```python
from build123d import *

# Parameters (mm, degrees)
PAD_DEPTH    = 39
PAD001_DEPTH = 35
SKETCH002_R  = 2.75
HOLE_DEPTH   = 10
HOLE_TIPS_R  = 2.75


with BuildPart() as part:
    # Sketch → Pad (new body)
    with BuildSketch(Plane.XZ):
        with BuildLine():
            ThreePointArc((8.810546, -10.5), (0, 13.706777), (-8.810546, -10.5))
            Line((-19.5, -10.5), (-8.810546, -10.5))
            Line((-19.5, -10.5), (-19.5, 8.5))
            Line((-19.5, 8.5), (-20.5, 8.5))
            Line((-20.5, 8.5), (-20.5, 17.5))
            Line((-20.5, 17.5), (-8.5, 17.5))
            Line((-8.5, 17.5), (-8.5, 16.5))
            Line((-8.5, 16.5), (8.5, 16.5))
            Line((8.5, 16.5), (8.5, 17.5))
            Line((8.5, 17.5), (20.5, 17.5))
            Line((20.5, 8.5), (20.5, 17.5))
            Line((19.5, 8.5), (20.5, 8.5))
            Line((19.5, -10.5), (19.5, 8.5))
            Line((8.810546, -10.5), (19.5, -10.5))
        make_face()
    extrude(amount=PAD_DEPTH)

    # Sketch001 (on DatumPlane) → Pad001 (join)
    with BuildSketch(Plane.XZ.offset(37)):
        with BuildLine():
            ThreePointArc((8.809308, -10.501039), (0.000808, 13.706777), (-8.810546, -10.5))
            Line((-7.713451, -9.192533), (-8.810546, -10.5))
            ThreePointArc((7.713451, -9.192533), (0, 12), (-7.713451, -9.192533))
            Line((7.713451, -9.192533), (8.809308, -10.501039))
        make_face()
    extrude(amount=-PAD001_DEPTH)

    # Sketch002 (on Face13 of Pad001) → Hole (cut)
    with BuildSketch(Plane(origin=(0, 0, 17.5), x_dir=(-1, 0, 0), z_dir=(0, 0, 1))):
        with Locations((-14, 32.5)):
            Circle(SKETCH002_R)
        with Locations((14, 32.5)):
            Circle(SKETCH002_R)
        with Locations((14, 6.5)):
            Circle(SKETCH002_R)
        with Locations((-14, 6.5)):
            Circle(SKETCH002_R)
    extrude(amount=-HOLE_DEPTH, mode=Mode.SUBTRACT)

    # Hole tips → Hole tip 1 section 0
    with BuildSketch(Plane(origin=(0, 0, 7.5), x_dir=(-1, 0, 0), z_dir=(0, 0, 1)), mode=Mode.PRIVATE) as hole_tip_1_s0:
        with Locations((-14, 32.5)):
            Circle(HOLE_TIPS_R)
    loft([hole_tip_1_s0.sketch, Vertex(14, -32.5, 5.847633)], mode=Mode.SUBTRACT)

    # Hole tips → Hole tip 2 section 0
    with BuildSketch(Plane(origin=(0, 0, 7.5), x_dir=(-1, 0, 0), z_dir=(0, 0, 1)), mode=Mode.PRIVATE) as hole_tip_2_s0:
        with Locations((14, 32.5)):
            Circle(HOLE_TIPS_R)
    loft([hole_tip_2_s0.sketch, Vertex(-14, -32.5, 5.847633)], mode=Mode.SUBTRACT)

    # Hole tips → Hole tip 3 section 0
    with BuildSketch(Plane(origin=(0, 0, 7.5), x_dir=(-1, 0, 0), z_dir=(0, 0, 1)), mode=Mode.PRIVATE) as hole_tip_3_s0:
        with Locations((14, 6.5)):
            Circle(HOLE_TIPS_R)
    loft([hole_tip_3_s0.sketch, Vertex(-14, -6.5, 5.847633)], mode=Mode.SUBTRACT)

    # Hole tips → Hole tip 4 section 0
    with BuildSketch(Plane(origin=(0, 0, 7.5), x_dir=(-1, 0, 0), z_dir=(0, 0, 1)), mode=Mode.PRIVATE) as hole_tip_4_s0:
        with Locations((-14, 6.5)):
            Circle(HOLE_TIPS_R)
    loft([hole_tip_4_s0.sketch, Vertex(14, -6.5, 5.847633)], mode=Mode.SUBTRACT)


solid = part.part
```
The model under review builds one solid part; all positions refer to its coordinate system, in mm. A direction names the side the tool comes from. Round coordinates to 2 decimals unless told otherwise and drop trailing zeros. Loops run counter-clockwise (first coordinate to the right, second up) from the corner with the lowest first, then second, coordinate; pieces in that order, holes last. Notation, with made-up numbers: M -25.5,54.25 L 14.5,54.25 A27 cw 14.5,78.25 Z; hole C -36.5,-38.75 d4. An arc over 180 degrees is marked long. Answer as a JSON object with one key per item and string values.
(1) Draft analysis for pull direction X (two halves, no side actions). For faces 1 (the flat face through (20.5, -19, 13)), 2 (the flat face through (8.254, -19.745, -9.838)), 3 (the flat face through (5, -39, 13)), 4 (the cylindrical face through (14.358, -35.227, 12.57)), state which applies: released by +X, released by -X, zero draft, split by the parting line, or undercut.
Resolved:
{"face 1": "released by +X", "face 2": "undercut", "face 3": "zero draft", "face 4": "undercut"}
(2) Tool access review of faces 5 (the flat face through (-20, -19, 8.5)), 6 (the flat face through (19.5, -19, -1)), 7 (the cylindrical face through (0.47, -0.99, 13.7)), 8 (the flat face through (8.5, -19, 17)), 9 (the cylindrical face through (-13.642, -35.227, 12.57)): name each direction out of +Z, -Z, +X, -X, +Y, -Y from which nothing blocks a thin tool from reaching the whole face with its end or side.
Resolved:
{"face 5": "-Z, -X, +Y, -Y", "face 6": "-Z, +X, +Y, -Y", "face 7": "+Y", "face 8": "+Z, +Y, -Y", "face 9": "+Z"}
(3) Clearance check with flat-ended pins moving along their axes: P1, Ø4, axis at x = 6, y = -8, coming from the -Z side; P2, Ø5, axis at x = 14, y = -6.5, coming from the +Z side; P3, Ø4.5, axis at x = -14, y = -6.5, coming from the +Z side. State where each tip first meets the part, or that it passes through.
Resolved:
{"P1": "z = -9.53", "P2": "z = 7.35", "P3": "z = 7.2"}
(4) To check wall thickness, follow line 1 along X through (y, z) = (-6.5, 14.75); line 2 along Y through (x, z) = (14, 10.75); line 3 along X through (y, z) = (-34, 0.5). State the ranges of each line that lie inside material, in increasing order.
Resolved:
{"line 1": "-20.5 to -16.75, -11.25 to 11.25, 16.75 to 20.5", "line 2": "-39 to -35.25, -29.75 to -9.25, -3.75 to 0", "line 3": "-19.5 to -11.99, 11.99 to 19.5"}
(5) Take a section at B-B on x = 0. Give the boundary of the cut face in (y, z).
Resolved:
{"outline": "M -39,13.71 L -37,13.71 L -37,12 L -2,12 L -2,13.71 L 0,13.71 L 0,16.5 L -39,16.5 Z"}
(6) Take a section at A-A on z = 0. Give the boundary of the cut face in (x, y), and give its area (3 significant figures).
Resolved:
{"outline": "M -19.5,-39 L -13.71,-39 L -13.71,-37 L -12,-37 L -12,-2 L -13.71,-2 L -13.71,0 L -19.5,0 Z; M 12,-37 L 13.71,-37 L 13.71,-39 L 19.5,-39 L 19.5,0 L 13.71,0 L 13.71,-2 L 12,-2 Z", "area": "571 mm²"}
(7) Take a section at D-D on z = -7.5. Give the boundary of the cut face in (x, y).
Resolved:
{"outline": "M -19.5,-39 L -11.47,-39 L -11.47,-37 L -9.37,-37 L -9.37,-2 L -11.47,-2 L -11.47,0 L -19.5,0 Z; M 9.37,-37 L 11.47,-37 L 11.47,-39 L 19.5,-39 L 19.5,0 L 11.47,0 L 11.47,-2 L 9.37,-2 Z"}
